The figure shows three views and two pictorial views of one solid part (mm, origin at its lowest corner). Answer the questions. Round coordinates to 2 decimals unless told otherwise and drop trailing zeros. Write each loop counter-clockwise with the first axis right and the second up, starting at its lowest first coordinate (ties: lowest second). Pieces come first, ordered by that corner, then holes.
Item 1: For a pull along X with two mould halves and no side action, classify the marked faces 1, 2 and 3 as +X half, -X half, draft (parallel to the pull), parting line (faces both ways), or undercut.
Item 2: Find the intervals of material crossed by probe 1 along X at (y, z) = (1.45, 3); probe 2 along X at (y, z) = (2.4, 1.75) (1 decimal); probe 3 along Z at (x, y) = (4, 1.8), in increasing order.
Item 3: Find section A-A on y = 1.45. Give the number of separate pieces and of enclosed holes in the cut face, then the cut area to 3 significant figures.
Item 4: Find section B-B on z = 2.65. Give the vertices of the cut face in (x, y), then the cut area to 3 significant figures.
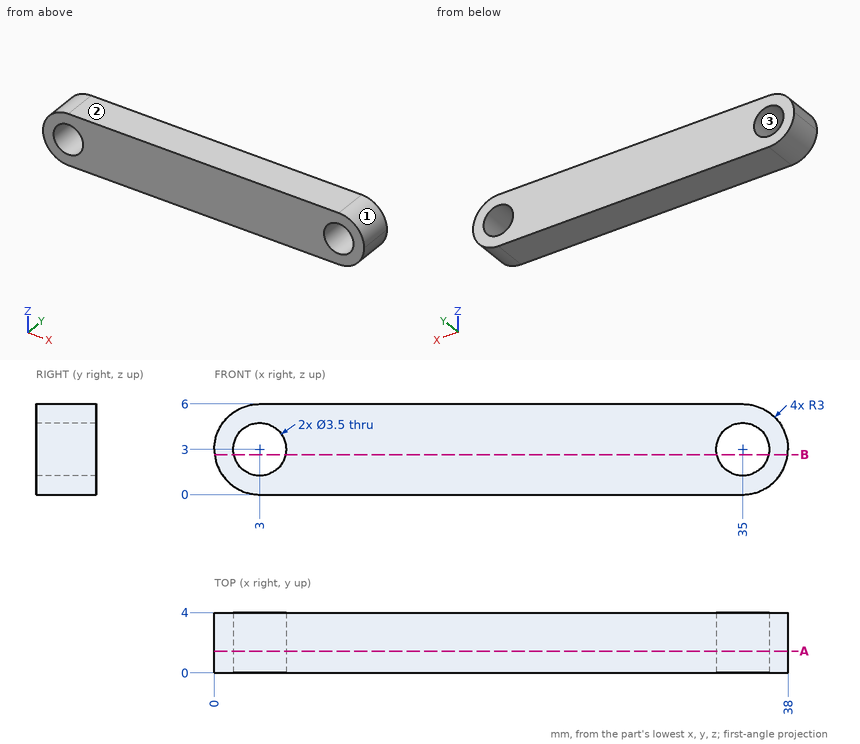
Check values:
1. face 1: +X half
1. face 2: draft
1. face 3: undercut
2. probe 1: x = 0 to 1.25, 4.75 to 33.25, 36.75 to 38
2. probe 2: x = 0.3 to 1.8, 4.2 to 33.8, 36.2 to 37.7
2. probe 3: z = 0 to 1.56, 4.44 to 6
3. separate pieces: 1
3. enclosed holes: 2
3. area: 201 mm2
4. outline: (0.02, 0) - (1.29, 0) - (1.29, 4) - (0.02, 4) - close; (4.71, 0) - (33.29, 0) - (33.29, 4) - (4.71, 4) - close; (36.71, 0) - (37.98, 0) - (37.98, 4) - (36.71, 4) - close
4. area: 124 mm2
